```python
from build123d import *

# Parameters (mm, degrees)
F0_R     = 40
F1_DEPTH = 50


with BuildPart() as f1:
    # F0 (on Front) → F1 (new body)
    with BuildSketch(Plane.XZ):
        with BuildLine():
            Line((-25, 250), (-25, 158.034806))
            ThreePointArc((-25, 158.034806), (-138.564065, 80), (-149.362157, -57.366768))
            Line((-149.362157, -57.366768), (-229.006351, -103.349365))
            Line((-229.006351, -103.349365), (-204.006351, -146.650635))
            Line((-204.006351, -146.650635), (-124.362157, -100.668038))
            ThreePointArc((-124.362157, -100.668038), (0, -160), (124.362157, -100.668038))
            Line((124.362157, -100.668038), (204.006351, -146.650635))
            Line((204.006351, -146.650635), (229.006351, -103.349365))
            Line((229.006351, -103.349365), (149.362157, -57.366768))
            ThreePointArc((149.362157, -57.366768), (138.564065, 80), (25, 158.034806))
            Line((25, 158.034806), (25, 250))
            Line((25, 250), (-25, 250))
        make_face()
        Circle(F0_R, mode=Mode.SUBTRACT)
    extrude(amount=-F1_DEPTH)


solid = f1.part
```
Here's how the part is built. I have some questions about the finished solid (model axes, mm). A direction names the side the tool comes from. Coordinates: 2 decimals unless noted, no trailing zeros. Write each loop counter-clockwise with the first axis right and the second up, starting at its lowest first coordinate (ties: lowest second). Pieces come first, ordered by that corner, then holes. Notation, with made-up numbers: (14.25, 36.5) - (25.25, 36.5) arc R16 cw to (25.25, 40.5) - close; hole circle Ø7 at (34, 44.5). An arc over 180 degrees is marked (long way). One line per item, written item: value.
1) On a 3-axis mill with a long thin cutter (end or side, diameter ignored), from which of +Z, -Z, +X, -X, +Y, -Y can I reach the whole of each face in a straight line? I mean faces 5 (the flat face through (25, 25, 203)), 6 (the flat face through (-25, 25, 205)), 7 (the flat face through (163.63, 24.65, -123.34)). Say none if no direction works.
Model answer:
face 5: +Z, +X, +Y, -Y
face 6: +Z, -X, +Y, -Y
face 7: -Z, +Y, -Y
2) I need wall thicknesses on line 1 along X through (y, z) = (41.5, -134); line 2 along X through (y, z) = (37.5, 198); line 3 along Z through (x, y) = (-34, 9.5). Which ranges of each line are inside material? Lowest first, please.
Model answer:
line 1: x = -211.31 to -182.09, -87.43 to 87.43, 182.09 to 211.31
line 2: x = -25 to 25
line 3: z = -156.35 to -21.07, 21.07 to 156.35
3) We'd pull the mould along X, two halves only. Please class faces 1 (the flat face through (-164.74, 24.65, -123.98)), 2 (the cylindrical face through (139.55, 24.65, 78.27)), 3 (the flat face through (-216.68, 24.65, -124.7)), 4 (the cylindrical face through (-1.994, 24.65, -159.988)): pulls with the +X half, pulls with the -X half, needs draft (parallel to the pull), parting line crosses it, or undercut.
Model answer:
face 1: undercut
face 2: pulls with the +X half
face 3: pulls with the -X half
face 4: undercut
4) Suppose I cut it at C-C on y = 23. Write out the boundary of the cut face in (x, z).
Model answer:
outline: (-229.01, -103.35) - (-204.01, -146.65) - (-124.36, -100.67) arc R160 ccw to (124.36, -100.67) - (204.01, -146.65) - (229.01, -103.35) - (149.36, -57.37) arc R160 ccw to (25, 158.03) - (25, 250) - (-25, 250) - (-25, 158.03) arc R160 ccw to (-149.36, -57.37) - close; hole circle Ø80 at (0, 0)
5) Suppose I cut it at B-B on x = 0. Write out the boundary of the cut face in (y, z), and give its area (3 significant figures).
Model answer:
outline: (0, -160) - (50, -160) - (50, -40) - (0, -40) - close; (0, 40) - (50, 40) - (50, 250) - (0, 250) - close
area: 16,500 mm²
6) Suppose I cut it at D-D on x = -115.5. Write out the boundary of the cut face in (y, z), and give its area (3 significant figures).
Model answer:
outline: (0, -110.72) - (50, -110.72) - (50, 110.72) - (0, 110.72) - close
area: 11,100 mm²
7) Suppose I cut it at A-A on z = 0. Write out the boundary of the cut face in (x, y), and give its area (3 significant figures).
Model answer:
outline: (-160, 0) - (-40, 0) - (-40, 50) - (-160, 50) - close; (40, 0) - (160, 0) - (160, 50) - (40, 50) - close
area: 12,000 mm²
8) I'm going to push flat-ended pins straight in: P1, Ø6, axis at x = -50, y = 35.5, coming from the -Z side; P2, Ø15, axis at y = 24, z = 189.5, coming from the -X side; P3, Ø3, axis at x = 48, y = 15.5, coming from the +Z side. Where does each tip first touch, or does it pass through?
Model answer:
P1: stops at z = -152.94
P2: stops at x = -25
P3: stops at z = 153.09
